Geometry: final body of the model. Coordinates: model frame, mm. A direction names the side the tool comes from. Give positions to 0.01 mm unless a question says otherwise; leave off trailing zeros. Order: outer loops, then holes, each group sorted by start corner. A loop starts at its lowest first (then second) coordinate and runs counter-clockwise, first axis right, second up. Notation, with made-up numbers: (54, 10.5) - (84, 10.5) arc R26 cw to (84, 32.5) - close; hole circle Ø10 at (72.5, 89.25). An arc over 180 degrees is marked (long way). Use one line per item in the form item = value.
from build123d import *

# Parameters (mm, degrees)
F1_DEPTH = 3
F3_DEPTH = 3
F4_W     = 19.5
F4_H     = 6.25
F5_DEPTH = 6


with BuildPart() as f1:
    # F0 (on Right) → F1 (new body, symmetric)
    with BuildSketch(Plane.YZ):
        Polygon((17, -26), (17, 0), (-17, 0), (-17, -28.974615), align=None)
    extrude(amount=F1_DEPTH, both=True)

    # F2 (on Right) → F3 (join, symmetric)
    with BuildSketch(Plane.YZ):
        Polygon((-17, -28.974615), (-16.477066, -34.951783), (-6.824001, -34.107249), (-7.346936, -28.130081), align=None)
        Polygon((17.522934, -31.977168), (17, -26), (7.346936, -26.844534), (7.86987, -32.821702), align=None)
    extrude(amount=F3_DEPTH, both=True)

    # F4 (on face) → F5 (cut, through all)
    with BuildSketch(Plane.YZ.offset(3)):
        with Locations((0, -6.125)):
            Rectangle(F4_W, F4_H)
    extrude(amount=-F5_DEPTH, mode=Mode.SUBTRACT)


solid = f1.part
(1) Contact query for flat-ended pins moving along their axis: pin 1 Ø3 at (x, z) = (0.5, -12.5) entering from +Y; pin 2 Ø1.5 at (x, y) = (2, -1) entering from -Z. Output: stop coordinate, or through.
Computed values:
pin_1 = 17
pin_2 = -27.64
(2) Ray query, line 1 along Y through (x, z) = (-2, -6.5); line 2 along Y through (x, z) = (2.5, -26); line 3 along Z through (x, y) = (-0.5, -9). Return the intervals inside material, ascending.
Computed values:
line_1 = -17 to -9.75, 9.75 to 17
line_2 = -17 to 17
line_3 = -34.3 to -9.25, -3 to 0
(3) Cut plane D-D on z = -25. Output: boundary loops of the cut face in (x, y), plus the area to 3 significant figures.
Computed values:
outline = (-3, -17) - (3, -17) - (3, 17) - (-3, 17) - close
area = 204 mm²
(4) Pull-direction query (Z, two-part tool) for faces 1 (the face through (0, -9.75, -6)), 2 (the face through (0, 0, 0)), 3 (the face through (0, -17, -14)); classes: released by +Z, released by -Z, zero draft, split by the parting line, or undercut.
Computed values:
face_1 = undercut
face_2 = released by +Z
face_3 = zero draft
(5) Cut plane C-C on x = 2.4. Output: boundary loops of the cut face in (y, z).
Computed values:
outline = (-17, -28.97) - (-16.48, -34.95) - (-6.82, -34.11) - (-7.35, -28.13) - (7.35, -26.84) - (7.87, -32.82) - (17.52, -31.98) - (17, -26) - (17, 0) - (-17, 0) - close; hole (-9.75, -9.25) - (9.75, -9.25) - (9.75, -3) - (-9.75, -3) - close
(6) Reachability of faces 4 (the face through (0, 17, -13)), 5 (the face through (0, 0, -9.25)), 6 (the face through (0.042, 7.605, -29.791)), 7 (the face through (0.042, 12.629, -32.405)) from +Z, -Z, +X, -X, +Y, -Y: full face, straight path, thin tool, end or side. Return the list, or none.
Computed values:
face_4 = +Z, +X, -X, +Y
face_5 = +X, -X
face_6 = -Z, +X, -X
face_7 = -Z, +X, -X, +Y
(7) Cut plane A-A on z = -8. Output: boundary loops of the cut face in (x, y), plus the area to 3 significant figures.
Computed values:
outline = (-3, -17) - (3, -17) - (3, -9.75) - (-3, -9.75) - close; (-3, 9.75) - (3, 9.75) - (3, 17) - (-3, 17) - close
area = 87.0 mm²
(8) Cut plane B-B on y = -0.5. Output: boundary loops of the cut face in (x, z).
Computed values:
outline = (-3, -27.53) - (3, -27.53) - (3, -9.25) - (-3, -9.25) - close; (-3, -3) - (3, -3) - (3, 0) - (-3, 0) - close
